Autodesk Fusion 360 part; units mm, degrees
sketch "Sketch1" plane through (0, 0, 0) normal (0, 1, 0) x (1, 0, 0)
  circle A0 centre (0, 0) radius 12.7
  circle A1 centre (0, 0) radius 9.525 construction
  circle A2 centre (-0.0005, 9.525) radius 1.55
  circle A3 centre (-8.2491, 4.7621) radius 1.55
  circle A4 centre (-8.2487, -4.7629) radius 1.55
  circle A5 centre (0.0005, -9.525) radius 1.55
  circle A6 centre (8.2491, -4.7621) radius 1.55
  circle A7 centre (8.2487, 4.7629) radius 1.55
  circle A8 centre (0, 0) radius 3
  dimension "d1" = 25.4
  dimension "d2" = 19.05
  dimension "d3" = 3.1
  dimension "d5" = 360
  dimension "d6" = 6
extrude "Extrude1" add sketch "Sketch1" along normal blind 5
Here's how the part is built. I have some questions about the finished solid (model axes, mm). Coordinates: 2 decimals unless noted, no trailing zeros. Order: outer loops, then holes, each group sorted by start corner. A loop starts at its lowest first (then second) coordinate and runs counter-clockwise, first axis right, second up.
1) Imagine slicing it at D-D on y = 4.1. State how many separate pieces and enclosed holes the cut face has, and give its area (3 significant figures).
2) Will these pins go through, and if not, where does the flat tip stop? pin 1 (5 mm diameter, centred on x = 8.25, z = 4.76, fed in from -Y); pin 2 (3 mm diameter, centred on x = 0, z = -9.52, fed in from +Y) (1 decimal); pin 3 (1.5 mm diameter, centred on y = 1, z = -6.5, fed in from +X); pin 4 (2 mm diameter, centred on x = -3, y = 0.5, fed in from +Z).
3) Imagine slicing it at B-B on x = 0. List the corners of the cut face in (y, z) for me (3 decimals), and give its area (3 significant figures).
4) We'd pull the mould along Z, two halves only. Please class faces 1 (the face through (-2.75, 2.46, -12.4)), 2 (the face through (3, 5, 3)), 3 (the face through (-3, 2, 0)): +Z half, -Z half, draft (parallel to the pull), parting line (faces both ways), or undercut.
5) I need wall thicknesses on line 1 (Z direction, x = -8.75, y = 4.75); line 2 (Z direction, x = -7.5, y = 0.7); line 3 (X direction, y = 2.55, z = 0). Which ranges of each line are inside material? Lowest first, please.
6) Imagine slicing it at A-A on z = 0. List the corners of the cut face in (x, y) for me.
7) Imagine slicing it at C-C on z = 4.25. List the corners of the cut face in (x, y) for me.
Response values:
1. separate pieces: 1
1. enclosed holes: 7
1. area: 433 mm2
2. pin 1: stops at y = 0
2. pin 2: passes through
2. pin 3: stops at x = 11.32
2. pin 4: stops at z = 12.54
3. outline: (0, -12.7) - (5, -12.7) - (5, -11.075) - (0, -11.075) - close; (0, -7.975) - (5, -7.975) - (5, -3) - (0, -3) - close; (0, 3) - (5, 3) - (5, 7.975) - (0, 7.975) - close; (0, 11.075) - (5, 11.075) - (5, 12.7) - (0, 12.7) - close
3. area: 66.0 mm2
4. face 1: parting line
4. face 2: draft
4. face 3: undercut
5. line 1: z = -9.2 to -6.23, -3.3 to 3.3, 6.23 to 9.2
5. line 2: z = -10.25 to -6.12, -3.41 to 3.41, 6.12 to 10.25
5. line 3: x = -12.7 to -3, 3 to 12.7
6. outline: (-12.7, 0) - (-3, 0) - (-3, 5) - (-12.7, 5) - close; (3, 0) - (12.7, 0) - (12.7, 5) - (3, 5) - close
7. outline: (-11.97, 0) - (-9.71, 0) - (-9.71, 5) - (-11.97, 5) - close; (-6.79, 0) - (6.79, 0) - (6.79, 5) - (-6.79, 5) - close; (9.71, 0) - (11.97, 0) - (11.97, 5) - (9.71, 5) - close
